Part print with two shaded views. Sizes in mm from the minimum x, y, z corner. Give positions to 0.01 mm unless a question says otherwise; leave off trailing zeros. Write each loop counter-clockwise with the first axis right and the second up, starting at its lowest first coordinate (ties: lowest second). Pieces come first, ordered by that corner, then holes. Notation, with made-up numbers: (-33, 29) - (-14, 29) arc R18 ccw to (-14, 62) - close; hole circle Ø2 at (26.25, 26.5). An arc over 180 degrees is marked (long way). Answer as a JSON object with one key per item and string values.
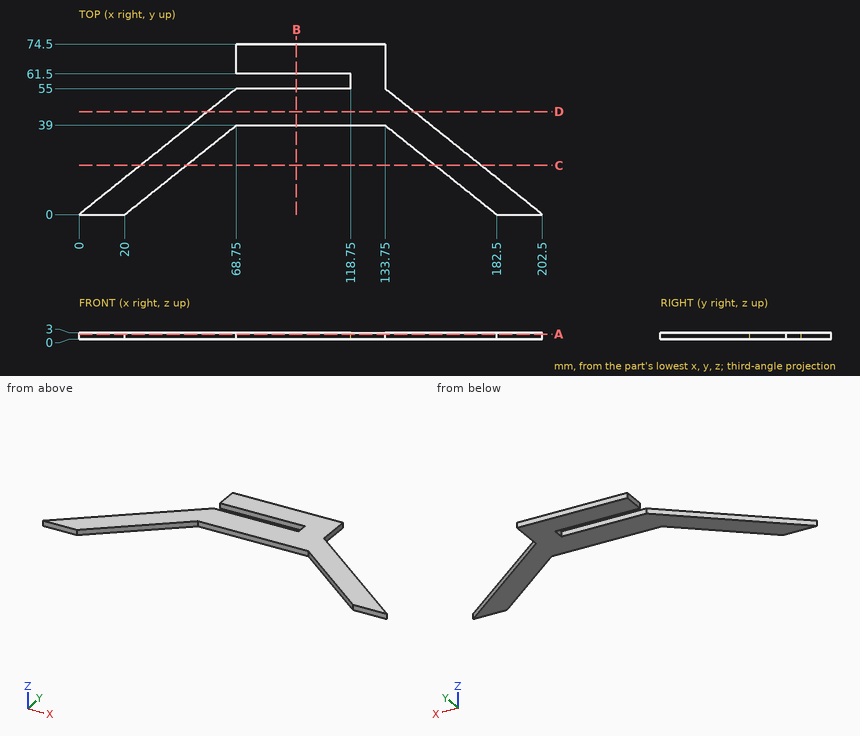
(1) Saw through at B-B, the plane x = 95. Give the cut face in (y, z), and give its area (3 significant figures).
Answer key:
{"outline": "(39, 0) - (55, 0) - (55, 3) - (39, 3) - close; (61.5, 0) - (74.5, 0) - (74.5, 3) - (61.5, 3) - close", "area": "87.0 mm²"}
(2) Probe L1, parallel to Y at x = 114, z = 0.65; L2, parallel to X at y = 60.5, z = 0.75; L3, parallel to X at y = 10, z = 2.65. List the from-to ranges inside material, lowest first. Write a range as [from, to].
Answer key:
{"L1": "y = [39, 55], [61.5, 74.5]", "L2": "x = [118.75, 133.75]", "L3": "x = [12.5, 32.5], [170, 190]"}
(3) Saw through at C-C, the plane y = 21.5. Give the cut face in (x, z) (3 decimals).
Answer key:
{"outline": "(26.875, 0) - (46.875, 0) - (46.875, 3) - (26.875, 3) - close; (155.625, 0) - (175.625, 0) - (175.625, 3) - (155.625, 3) - close"}
(4) Saw through at D-D, the plane y = 45. Give the cut face in (x, z).
Answer key:
{"outline": "(56.25, 0) - (146.25, 0) - (146.25, 3) - (56.25, 3) - close"}
(5) Flat gauge pins, fed straight in: P1, Ø0.9, axis at x = 100, z = 2, coming from the -Y side; P2, Ø0.9, axis at y = 67.5, z = 1.5, coming from the -X side; P3, Ø0.9, axis at y = 61.5, z = 2, coming from the +X side. Where does each tip first touch, or does it go through?
Answer key:
{"P1": "stops at y = 39", "P2": "stops at x = 68.75", "P3": "stops at x = 133.75"}
(6) Saw through at A-A, the plane z = 2.35. Give the cut face in (x, y).
Answer key:
{"outline": "(0, 0) - (20, 0) - (68.75, 39) - (133.75, 39) - (182.5, 0) - (202.5, 0) - (133.75, 55) - (133.75, 74.5) - (68.75, 74.5) - (68.75, 61.5) - (118.75, 61.5) - (118.75, 55) - (68.75, 55) - close"}
